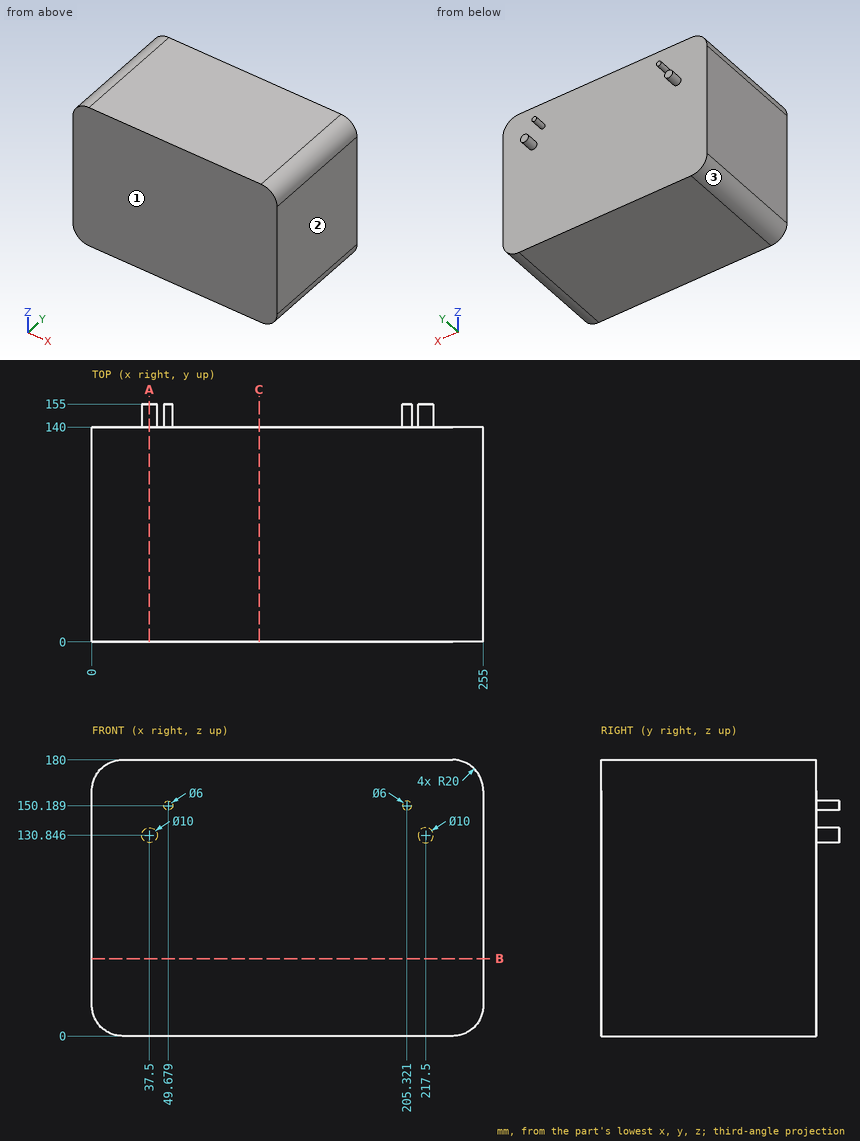
Could you check a few things on this drawing? It's one solid part, dimensions in mm from its lowest x, y, z. Give positions to 0.01 mm unless a question says otherwise; leave off trailing zeros. Write each loop counter-clockwise with the first axis right and the second up, starting at its lowest first coordinate (ties: lowest second). Pieces come first, ordered by that corner, then holes. Notation, with made-up numbers: M -25.75,2.5 L 12.25,2.5 A23 ccw 12.25,29.5 Z; hole C 76.25,6.25 d4. An arc over 180 degrees is marked long. Put each result on its own line as item: value. Start each with the question number.
Item 1: If we section it at C-C, the plane x = 109: Write out the boundary of the cut face in (y, z), then the cut area to 3 significant figures.
Item 2: Will this pin go through, and if not, where does the flat tip stop? pin 1 (10 mm diameter, centred on x = 27, z = 73.5, fed in from +Y).
Item 3: If we section it at A-A, the plane x = 37.5: Write out the boundary of the cut face in (y, z), then the cut area to 4 significant figures.
Item 4: If we section it at B-B, the plane z = 50.5: Write out the boundary of the cut face in (x, y).
Item 5: I need wall thicknesses on L1, parallel to Y at x = 110, z = 26.5; L2, parallel to X at y = 29.5, z = 12; L3, parallel to Z at x = 13, y = 28 (1 decimal). Which ranges of each line are inside material? Lowest first, please. Write a range as from..to.
Item 6: Thinking about a two-plate mould opening in X: for the marked faces 1, 2 and 3, which applies, +X half, -X half, draft (parallel to the pull), parting line (faces both ways), or undercut?
Values:
1. outline: M 0,0 L 140,0 L 140,180 L 0,180 Z
1. area: 25,200 mm²
2. pin 1: y = 140
3. outline: M 0,0 L 140,0 L 140,125.85 L 155,125.85 L 155,135.85 L 140,135.85 L 140,180 L 0,180 Z
3. area: 25,350 mm²
4. outline: M 0,0 L 255,0 L 255,140 L 0,140 Z
5. L1: 0..140
5. L2: 1.67..253.33
5. L3: 1.3..178.7
6. face 1: draft
6. face 2: +X half
6. face 3: -X half
